```python
from build123d import *

# Parameters (mm, degrees)
SKETCH_1_R      = 28
SKETCH_1_R_2    = 25
EXTRUDE_1_DEPTH = 100
SKETCH_2_R      = 30
EXTRUDE_2_DEPTH = 5


with BuildPart() as part:
    # 草图1 → 凸台-拉伸1 (new body)
    with BuildSketch(Plane(origin=(0, 0, 0), x_dir=(1, 0, 0), z_dir=(0, 1, 0))):
        with Locations(Location((0, 0, 0), (0, 0, 270))):
            Circle(SKETCH_1_R)
        with Locations(Location((0, 0, 0), (0, 0, 270))):
            Circle(SKETCH_1_R_2, mode=Mode.SUBTRACT)
    extrude(amount=EXTRUDE_1_DEPTH)

    # 草图2 → 凸台-拉伸2 (add)
    with BuildSketch(Plane.XZ):
        with Locations(Location((0, 0, 0), (0, 0, 270))):
            Circle(SKETCH_2_R)
    extrude(amount=EXTRUDE_2_DEPTH)

    # 倒角3: read off the stored shape, not the designer's step
    # 倒角3 outline → 倒角3 (revolve, cut)
    with BuildSketch(Plane.XY):
        Polygon((30, 0), (28, 0), (30, -5), align=None)
    revolve(axis=Axis((0, 0, 0), (0, 1, 0)), mode=Mode.SUBTRACT)


solid = part.part
```
Read the model definition and answer for the solid it produces. Units are mm, in the model's axes. A direction names the side the tool comes from. Round coordinates to 2 decimals unless told otherwise and drop trailing zeros. Loops run counter-clockwise (first coordinate to the right, second up) from the corner with the lowest first, then second, coordinate; pieces in that order, holes last. Notation, with made-up numbers: (77.25, 30) -> (128.25, 30) arc R16 cw to (128.25, 60) -> close; hole circle Ø8 at (-15.5, 87.5). An arc over 180 degrees is marked (long way). One line per item, written item: value.
1) Consider L1, parallel to X at y = 29, z = 0; L2, parallel to X at y = 82, z = -4.5; L3, parallel to Y at x = 17.5, z = -13. Determine where each line is inside the solid, lowest interval first. Write a range as [from, to].
Answer list:
L1: x = [-28, -25], [25, 28]
L2: x = [-27.64, -24.59], [24.59, 27.64]
L3: y = [-5, 0]
2) A cutting plane is placed at B-B (x = 0). Determine the outline of the cut face in (y, z), and give its area (3 significant figures).
Answer list:
outline: (-5, -30) -> (0, -28) -> (100, -28) -> (100, -25) -> (0, -25) -> (0, 25) -> (100, 25) -> (100, 28) -> (0, 28) -> (-5, 30) -> close
area: 890 mm²
3) Flat-ended cylindrical pins translate along their axes: P1, Ø5, axis at x = 18.5, y = 47, coming from the +Z side; P2, Ø12, axis at y = 43, z = 21.5, coming from the -X side; P3, Ø8, axis at y = 48, z = 21.5, coming from the +X side. Find the tip coordinate at first contact, or state that the pin passes through.
Answer list:
P1: stops at z = 22.98
P2: stops at x = -23.32
P3: stops at x = 21.86
4) For faces 4 (the face through (0, -5, 0)), 5 (the face through (7.509, 49.3, 23.846)), determine the directions among +Z, -Z, +X, -X, +Y, -Y from which every point of the face is accessible in a straight line to the end or side of a thin tool.
Answer list:
face 4: +Z, -Z, +X, -X, -Y
face 5: +Y
5) The mould has two halves that part along Z. Classify faces 1 (the face through (0, 0, 0)), 2 (the face through (23, 100, -11)), 3 (the face through (-27.334, 49.3, -6.07)): pulls with the +Z half, pulls with the -Z half, needs draft (parallel to the pull), parting line crosses it, or undercut.
Answer list:
face 1: undercut
face 2: needs draft
face 3: parting line crosses it
6) A cutting plane is placed at A-A (y = 34). Determine the outline of the cut face in (x, z), and give its area (3 significant figures).
Answer list:
outline: circle Ø56 at (0, 0); hole circle Ø50 at (0, 0)
area: 500 mm²
7) A cutting plane is placed at C-C (z = 0). Determine the outline of the cut face in (x, y), and give its area (3 significant figures).
Answer list:
outline: (-30, -5) -> (30, -5) -> (28, 0) -> (28, 100) -> (25, 100) -> (25, 0) -> (-25, 0) -> (-25, 100) -> (-28, 100) -> (-28, 0) -> close
area: 890 mm²
